Can you work these out from the model? Positions are in its coordinate system, mm. A direction names the side the tool comes from. Give positions to 0.01 mm unless a question says otherwise; leave off trailing zeros. Loops run counter-clockwise (first coordinate to the right, second up) from the corner with the lowest first, then second, coordinate; pieces in that order, holes last. Notation, with made-up numbers: M 4.25,-15 L 50.25,-15 A22 cw 50.25,22 Z; hole C -21,-1 d6. An arc over 180 degrees is marked long. One line per item, written item: value. Start each with the question number.
Autodesk Inventor part; units mm, degrees
ref_plane "YZ Plane" through (0, 0, 0) normal (1, 0, 0) x (0, 1, 0)
ref_plane "XZ Plane" through (0, 0, 0) normal (0, 1, 0) x (-1, 0, 0)
ref_plane "XY Plane" through (0, 0, 0) normal (0, 0, 1) x (1, 0, 0)
sketch "草圖1" plane through (0, 0, 0) normal (0, 0, 1) x (1, 0, 0)
  line L0 (0, 0) -> (51.3, 0)
  line L1 (51.3, 0) -> (51.3, 36.8)
  line L2 (51.3, 36.8) -> (38.5, 36.8)
  line L3 (38.5, 36.8) -> (14.22, 71.58)
  line L4 (14.22, 71.58) -> (0, 71.58)
  line L5 (0, 71.58) -> (0, 50.64)
  line L6 (0, 50.64) -> (14.22, 50.64)
  line L7 (14.22, 50.64) -> (14.22, 36.8)
  line L8 (14.22, 36.8) -> (0, 36.8)
  line L9 (0, 0) -> (0, 36.8)
  dimension "d0" = 36.8
  dimension "d1" = 14.22
  dimension "d3" = 13.84
  dimension "d4" = 14.22
  dimension "d5" = 71.58
  dimension "d6" = 51.3
  dimension "d7" = 12.8
extrude "擠出1" add sketch "草圖1" along normal blind 51.2
sketch "草圖2" plane through (0, 0, 0) normal (-1, 0, 0) x (0, 0, 1)
  line L0 (0, 0) -> (51.2, 0)
  line L1 (12.1, 0) -> (12.1, 25.5)
  line L2 (12.1, 25.5) -> (37.8, 25.5)
  line L3 (37.8, 25.5) -> (37.8, -6.925)
  line L4 (37.8, -6.925) -> (13.9148, -5.9857)
  line L5 (13.9148, -5.9857) -> (12.1, 0)
  line L6 (51.2, 36.8) -> (51.2, 0)
  dimension "d10" = 25.7
  dimension "d12" = 13.4
  dimension "d13" = 25.5
extrude "擠出2" cut sketch "草圖2" against normal up to next
sketch "草圖3" plane through (0, 0, 51.2) normal (0, -1, 0) x (1, 0, 0)
  circle A0 centre (44.3, -7.4) radius 2.5
  line L0 (0, -13.4) -> (51.3, -13.4)
  line L1 (51.3, -13.4) -> (51.3, 0)
  circle A1 centre (5.9, -7.4) radius 2.5
  point P0 (0, -51.2)
  dimension "d16" = 5
  dimension "d18" = 6
  dimension "d19" = 7
  dimension "d22" = 38.4
extrude "擠出3" cut sketch "草圖3" against normal blind 12.5
pattern_linear "矩形陣列1" count 2 spacing 39 along (0, 0, -1) of "擠出3"
properties part number "小虎鉗-左側" material "鋁合金 6061"
Q1. If we section it at A-A, the plane x = 5.9: Write out the boundary of the cut face in (y, z).
Q2. For P1, Ø2, axis at y = 8.5, z = 45, coming from the -X side; P2, Ø4, axis at x = 44.5, z = 43.5, coming from the -Y side; P3, Ø3, axis at y = 62.5, z = 27, coming from the +X side; P4, Ø4, axis at x = 6.5, z = 20.5, coming from the -Y side, each with a flat end and sliding along its axis, tell me the tip position at first contact or that it passes through.
Q3. I need wall thicknesses on line 1 along Z through (x, y) = (5.9, 9.5); line 2 along Z through (x, y) = (5, 7); line 3 along Y through (x, z) = (8, 37). Which ranges of each line are inside material? Lowest first, please.
Q4. Which directions (+Z, -Z, +X, -X, +Y, -Y) give clear straight access to the entire face, cutting with the end or side of a thin tool? Please do faces 1 (the face through (7, 36.8, 25)), 2 (the face through (44, 12.5, 5)), 3 (the face through (25, 0, 6)), 4 (the face through (25, 13, 12.1)), 5 (the face through (51.3, 26, 25)).
Q5. If we mould it in two halves opening along Z, with no side actions, what happens to faces 6 (the face through (25, 28, 0)), 7 (the face through (7, 71.58, 25)), 8 (the face through (3.9, 6.2, 3.3)), 9 (the face through (41.8, 6.2, 4.9))? For each: released by +Z, released by -Z, zero draft, split by the parting line, or undercut.
Q6. If we section it at B-B, the plane z = 17: Write out the boundary of the cut face in (x, y).
Q7. If we section it at C-C, the plane x = 44.3: Write out the boundary of the cut face in (y, z).
Q8. If we section it at D-D, the plane z = 4.8: Write out the boundary of the cut face in (x, y), plus the area to 3 significant figures.
Response:
1. outline: M 0,0 L 36.8,0 L 36.8,51.2 L 0,51.2 L 0,46.3 L 12.5,46.3 L 12.5,41.3 L 0,41.3 L 0,37.8 L 25.5,37.8 L 25.5,12.1 L 0,12.1 L 0,7.3 L 12.5,7.3 L 12.5,2.3 L 0,2.3 Z; M 50.64,0 L 71.58,0 L 71.58,51.2 L 50.64,51.2 Z
2. P1: x = 0
2. P2: y = 12.5
2. P3: x = 21.61
2. P4: y = 25.5
3. line 1: 0 to 2.3, 7.3 to 12.1, 37.8 to 41.3, 46.3 to 51.2
3. line 2: 0 to 2.47, 7.13 to 12.1, 37.8 to 41.47, 46.13 to 51.2
3. line 3: 25.5 to 36.8, 50.64 to 71.58
4. face 1: +Z, -Z, -X
4. face 2: -Y
4. face 3: +Z, -Z, +X, -X, -Y
4. face 4: +X, -X, -Y
4. face 5: +Z, -Z, +X, +Y, -Y
5. face 6: released by -Z
5. face 7: zero draft
5. face 8: undercut
5. face 9: undercut
6. outline: M 0,25.5 L 51.3,25.5 L 51.3,36.8 L 38.5,36.8 L 14.22,71.58 L 0,71.58 L 0,50.64 L 14.22,50.64 L 14.22,36.8 L 0,36.8 Z
7. outline: M 0,0 L 36.8,0 L 36.8,51.2 L 0,51.2 L 0,46.3 L 12.5,46.3 L 12.5,41.3 L 0,41.3 L 0,37.8 L 25.5,37.8 L 25.5,12.1 L 0,12.1 L 0,7.3 L 12.5,7.3 L 12.5,2.3 L 0,2.3 Z
8. outline: M 0,0 L 3.4,0 L 3.4,12.5 L 8.4,12.5 L 8.4,0 L 41.8,0 L 41.8,12.5 L 46.8,12.5 L 46.8,0 L 51.3,0 L 51.3,36.8 L 38.5,36.8 L 14.22,71.58 L 0,71.58 L 0,50.64 L 14.22,50.64 L 14.22,36.8 L 0,36.8 Z
8. area: 2,480 mm^2
